The listing builds one solid part. Answer for the finished solid, in the listing's coordinates (mm). Face numbers are marked on the shaded views. A direction names the side the tool comes from. Round coordinates to 2 decimals unless told otherwise and drop trailing zeros. Write each loop counter-clockwise with the first axis right and the second up, starting at its lowest first coordinate (ties: lowest second). Pieces come first, ordered by that corner, then holes. Notation, with made-up numbers: (-21.75, 26.25) - (36.25, 26.25) arc R18 cw to (36.25, 52.25) - close; hole circle Ø3 at (-22, -34). An arc over 180 degrees is marked (long way). Answer as CSV lines item,"result". Start each with the question number.
Item 1: Straight lines are drawn through the part: line 1 along Z through (x, y) = (0, 2); line 2 along Z through (x, y) = (3.75, -8.25); line 3 along Y through (x, z) = (-2, 3). For each, find the intervals that lie inside material, in ascending order. Write a range as [from, to].
Item 2: For a pull along Z with two mould halves and no side action, classify the marked faces 1, 2 and 3 as pulls with the +Z half, pulls with the -Z half, needs draft (parallel to the pull), parting line crosses it, or undercut.
Item 3: A cutting plane is placed at A-A on x = -10. Determine the outline of the cut face in (y, z).
Item 4: Which of the six approach directions +Z, -Z, +X, -X, +Y, -Y give full straight-line access (tool end or side, diameter ignored) to the marked faces 4, 5, 6, 7 and 8?
Item 5: Flat-ended cylindrical pins translate along their axes: pin 1 (5 mm diameter, centred on x = 1.5, z = 5, fed in from +Y); pin 2 (4.5 mm diameter, centred on y = 1.5, z = 7, fed in from -X); pin 3 (5 mm diameter, centred on x = 4, z = 7.5, fed in from -Y); pin 4 (2.5 mm diameter, centred on x = 10, y = 0, fed in from +Z). Find the tip coordinate at first contact, or state that the pin passes through.
Item 6: A cutting plane is placed at D-D on x = 0. Determine the outline of the cut face in (y, z) (3 decimals), and give its area (3 significant figures).
Item 7: A cutting plane is placed at C-C on x = -5. Determine the outline of the cut face in (y, z), and give its area (3 significant figures).
Item 8: A cutting plane is placed at B-B on y = -3. Determine the outline of the cut face in (x, z), and give its area (3 significant figures).
```python
from build123d import *

# Parameters (mm, degrees)
F0_R        = 15
F1_DEPTH    = 2
F2_W        = 12
F2_H        = 10
F3_DEPTH    = 10
F4_R        = 4.05
F5_DEPTH    = 20.001
F6_R        = 1.5
F7_DEPTH    = 2.001
F8_T1_DEPTH = 10
F8_T3_DEPTH = 14.5
F8_T5_DEPTH = 12.5


# Not quite as in the source:
# - a fillet or chamfer that OpenCascade refuses, or shapes differently, is made with other operations: its cross-section is extruded or revolved along the edge and cut away or added


with BuildPart() as f1:
    # F0 (on Top) → F1 (new body)
    with BuildSketch(Plane.XY):
        Circle(F0_R)
    extrude(amount=F1_DEPTH)

    # F2 (on face) → F3 (join)
    with BuildSketch(Plane.XY.offset(2)):
        Rectangle(F2_W, F2_H)
    extrude(amount=F3_DEPTH)

    # F4 (on face) → F5 (cut, through all)
    with BuildSketch(Plane.XZ.offset(5)):
        with Locations((0, 7)):
            Circle(F4_R)
    extrude(amount=-F5_DEPTH, mode=Mode.SUBTRACT)

    # F6 (on face) → F7 (cut, through all)
    with BuildSketch(Plane.XY.offset(2)):
        with Locations((10, 0)):
            Circle(F6_R)
        with Locations((-10, 0)):
            Circle(F6_R)
    extrude(amount=-F7_DEPTH, mode=Mode.SUBTRACT)

    # F8: fillet of radius 0.5 on 8 edges, made by hand

    # F8_s2 → F8_t1 (join)
    with BuildSketch(Plane.XZ.offset(-5)):
        with BuildLine():
            ThreePointArc((-6.5, 2), (-6.1464466094, 2.1464466094), (-6, 2.5))
            Line((-6, 2.5), (-6, 2))
            Line((-6, 2), (-6.5, 2))
        make_face()
        with BuildLine():
            ThreePointArc((6.5, 2), (6.1464466094, 2.1464466094), (6, 2.5))
            Line((6, 2.5), (6, 2))
            Line((6, 2), (6.5, 2))
        make_face()
    extrude(amount=F8_T1_DEPTH)

    # F8_s4 → F8_t3 (cut)
    with BuildSketch(Plane.YZ.offset(-7.25)):
        with BuildLine():
            ThreePointArc((-4.5, 12), (-4.8535533906, 11.8535533906), (-5, 11.5))
            Line((-5, 11.5), (-5, 12))
            Line((-5, 12), (-4.5, 12))
        make_face()
        with BuildLine():
            ThreePointArc((4.5, 12), (4.8535533906, 11.8535533906), (5, 11.5))
            Line((5, 11.5), (5, 12))
            Line((5, 12), (4.5, 12))
        make_face()
    extrude(amount=F8_T3_DEPTH, mode=Mode.SUBTRACT)

    # F8_s6 → F8_t5 (cut)
    with BuildSketch(Plane.XZ.offset(-6.25)):
        with BuildLine():
            ThreePointArc((5.5, 12), (5.8535533906, 11.8535533906), (6, 11.5))
            Line((6, 11.5), (6, 12))
            Line((6, 12), (5.5, 12))
        make_face()
        with BuildLine():
            ThreePointArc((-6, 11.5), (-5.8535533906, 11.8535533906), (-5.5, 12))
            Line((-5.5, 12), (-6, 12))
            Line((-6, 12), (-6, 11.5))
        make_face()
    extrude(amount=F8_T5_DEPTH, mode=Mode.SUBTRACT)

    # F8_s7 → F8_t8 (revolve, cut)
    with BuildSketch(Plane.XY.offset(7)):
        with BuildLine():
            ThreePointArc((4.05, 4.5), (4.1964466094, 4.8535533906), (4.55, 5))
            Line((4.55, 5), (4.05, 5))
            Line((4.05, 5), (4.05, 4.5))
        make_face()
    revolve(axis=Axis((0, 5, 7), (0, -1, 0)), mode=Mode.SUBTRACT)

    # F8_s9 → F8_t10 (revolve, cut)
    with BuildSketch(Plane.XY.offset(7)):
        with BuildLine():
            ThreePointArc((4.55, -5), (4.1964466094, -4.8535533906), (4.05, -4.5))
            Line((4.05, -4.5), (4.05, -5))
            Line((4.05, -5), (4.55, -5))
        make_face()
    revolve(axis=Axis((0, -5, 7), (0, -1, 0)), mode=Mode.SUBTRACT)


solid = f1.part
```
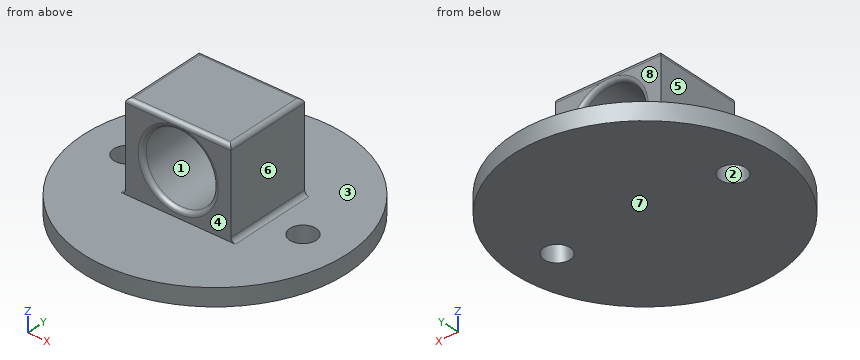
Geometry says:
1,line 1,"z = [0, 2.95], [11.05, 12]"
1,line 2,"z = [0, 2]"
1,line 3,"y = [-4.99, 4.99]"
2,face 1,"undercut"
2,face 2,"needs draft"
2,face 3,"pulls with the +Z half"
3,outline,"(-11.18, 0) - (-1.5, 0) - (-1.5, 2) - (-11.18, 2) - close; (1.5, 0) - (11.18, 0) - (11.18, 2) - (1.5, 2) - close"
4,face 4,"+Z, +X, -X, -Y"
4,face 5,"+Z, -X, +Y, -Y"
4,face 6,"+Z, +X, +Y, -Y"
4,face 7,"-Z, +X, -X, +Y, -Y"
4,face 8,"+Z, +X, -X, +Y"
5,pin 1,"stops at y = 5"
5,pin 2,"stops at x = -6"
5,pin 3,"stops at y = -5"
5,pin 4,"passes through"
6,outline,"(-15, 0) - (15, 0) - (15, 2) - (5, 2) - (5, 2.45) arc R0.5 ccw to (4.5, 2.95) - (-4.5, 2.95) arc R0.5 ccw to (-5, 2.45) - (-5, 2) - (-15, 2) - close; (-4.999, 11.525) arc R0.5 ccw to (-4.5, 11.05) - (4.5, 11.05) arc R0.5 ccw to (4.999, 11.525) arc R0.5 ccw to (4.5, 12) - (-4.5, 12) arc R0.5 ccw to start"
6,area,"78.7 mm^2"
7,outline,"(-14.14, 0) - (14.14, 0) - (14.14, 2) - (5, 2) - (5, 11.5) arc R0.5 ccw to (4.5, 12) - (-4.5, 12) arc R0.5 ccw to (-5, 11.5) - (-5, 2) - (-14.14, 2) - close"
7,area,"156 mm^2"
8,outline,"(-14.7, 0) - (14.7, 0) - (14.7, 2) - (6.5, 2) arc R0.5 cw to (6, 2.5) - (6, 11.5) arc R0.5 ccw to (5.5, 12) - (-5.5, 12) arc R0.5 ccw to (-6, 11.5) - (-6, 2.5) arc R0.5 cw to (-6.5, 2) - (-14.7, 2) - close; hole circle Ø8.1 at (0, 7)"
8,area,"127 mm^2"
